from build123d import *

# Parameters (mm, degrees)
ESBO_O1_W                                         = 40
ESBO_O1_H                                         = 38
RESSALTO_EXTRUS_O1_DEPTH                          = 8
ESBO_O2_R                                         = 11
CORTE_EXTRUS_O1_DEPTH                             = 9
FURO_ROSCADO_PARA_CONDU_TE_DE_M3X0_51_D           = 3.15
FURO_ROSCADO_PARA_CONDU_TE_DE_M3X0_51_DEPTH       = 10
FURO_ROSCADO_PARA_CONDU_TE_DE_M3X0_51_CSINK_D     = 3.766
FURO_ROSCADO_PARA_CONDU_TE_DE_M3X0_51_CSINK_ANGLE = 90
FURO_ROSCADO_PARA_CONDU_TE_DE_M3X0_51_TIP         = 0.946355475


with BuildPart() as part:
    # Esboço1 → Ressalto-extrusão1 (new body)
    with BuildSketch(Plane.XY):
        Rectangle(ESBO_O1_W, ESBO_O1_H)
    extrude(amount=RESSALTO_EXTRUS_O1_DEPTH)

    # Esboço2 → Corte-extrusão1 (cut, through all)
    with BuildSketch(Plane.XY.offset(8)):
        with Locations((0, 4.5)):
            Circle(ESBO_O2_R)
    extrude(amount=-CORTE_EXTRUS_O1_DEPTH, mode=Mode.SUBTRACT)

    # Furo roscado para conduíte de M3x0.51
    with Locations(Plane(origin=(0, -19, 0), x_dir=(-1, 0, 0), z_dir=(0, -1, 0))):
        with Locations((-12, -4), (12, -4)):
            CounterSinkHole(FURO_ROSCADO_PARA_CONDU_TE_DE_M3X0_51_D / 2, FURO_ROSCADO_PARA_CONDU_TE_DE_M3X0_51_CSINK_D / 2, depth=FURO_ROSCADO_PARA_CONDU_TE_DE_M3X0_51_DEPTH, counter_sink_angle=FURO_ROSCADO_PARA_CONDU_TE_DE_M3X0_51_CSINK_ANGLE)
            with Locations((0, 0, -(FURO_ROSCADO_PARA_CONDU_TE_DE_M3X0_51_DEPTH + FURO_ROSCADO_PARA_CONDU_TE_DE_M3X0_51_TIP / 2))):  # 118° drill point
                Cone(0, FURO_ROSCADO_PARA_CONDU_TE_DE_M3X0_51_D / 2, FURO_ROSCADO_PARA_CONDU_TE_DE_M3X0_51_TIP, mode=Mode.SUBTRACT)


solid = part.part
Geometry: final body of the model. Coordinates: model frame, mm. A direction names the side the tool comes from. Give positions to 0.01 mm unless a question says otherwise; leave off trailing zeros. Write each loop counter-clockwise with the first axis right and the second up, starting at its lowest first coordinate (ties: lowest second). Pieces come first, ordered by that corner, then holes. Notation, with made-up numbers: M 12.5,24 L 63.5,24 A17 ccw 63.5,40 Z; hole C 5,-5 d7. An arc over 180 degrees is marked long. Answer in a Markdown table with one row per item. Add a question column.
(1) Section A-A on y = 4.5. Return loops of the section in (x, z), and give its area (3 significant figures).
(2) Mould query, pull axis X, two halves, no side actions, for faces 1 (the cylindrical face through (-12.21, -13.78, 2.44)), 2 (the flat face through (0, -8, 0)), 3 (the flat face through (-20, 0, 4)). Classes: +X half, -X half, draft (parallel to the pull), parting line (faces both ways), or undercut.
(3) Reachability of faces 4 (the flat face through (0, -8, 8)), 5 (the cylindrical face through (11.79, -13.78, 2.44)) from +Z, -Z, +X, -X, +Y, -Y: full face, straight path, thin tool, end or side. Return the list, or none.
(4) Ray query, line 1 (X direction, y = -15.25, z = 4) (3 decimals); line 2 (Z direction, x = -12, y = -13.25) (3 decimals); line 3 (X direction, y = 8, z = 6.5). Return the intervals inside material, ascending.
(5) First-contact query: pin 1 (2.5 mm diameter, centred on x = -12, z = 4, fed in from -Y). Flat tip, straight axial feed; report the tip coordinate or a pass-through.
(6) Section B-B on x = 0. Return loops of the section in (y, z), and give its area (3 significant figures).
Result set:
| question | item | result |
|---|---|---|
| 1 | outline | M -20,0 L -11,0 L -11,8 L -20,8 Z; M 11,0 L 20,0 L 20,8 L 11,8 Z |
| 1 | area | 144 mm^2 |
| 2 | face 1 | undercut |
| 2 | face 2 | draft |
| 2 | face 3 | -X half |
| 3 | face 4 | +Z, +X, -X, +Y, -Y |
| 3 | face 5 | -Y |
| 4 | line 1 | x = -20 to -13.575, -10.425 to 10.425, 13.575 to 20 |
| 4 | line 2 | z = 0 to 2.425, 5.575 to 8 |
| 4 | line 3 | x = -20 to -10.43, 10.43 to 20 |
| 5 | pin 1 | stops at y = -8.8 |
| 6 | outline | M -19,0 L -6.5,0 L -6.5,8 L -19,8 Z; M 15.5,0 L 19,0 L 19,8 L 15.5,8 Z |
| 6 | area | 128 mm^2 |
